Autodesk Inventor part; units mm, degrees
ref_plane "YZ Plane" through (0, 0, 0) normal (1, 0, 0) x (0, 1, 0)
ref_plane "XZ Plane" through (0, 0, 0) normal (0, 1, 0) x (-1, 0, 0)
ref_plane "XY Plane" through (0, 0, 0) normal (0, 0, 1) x (1, 0, 0)
sketch "スケッチ1" plane through (0, 0, 0) normal (0, 0, 1) x (1, 0, 0)
  line L0 (0, 0) -> (0, 3)
  line L1 (0, 3) -> (0.2, 3)
  line L2 (0.2, 3) -> (1.7, 1.5)
  line L3 (1.7, 1.5) -> (7.7, 1.5)
  line L4 (7.7, 1.5) -> (7.7, 0)
  line L5 (0, 0) -> (7.7, 0)
  dimension "d0" = 45
  dimension "d1" = 3
  dimension "d2" = 1.7
  dimension "d3" = 1.5
  dimension "d4" = 6
revolve "回転1" add sketch "スケッチ1" angle 360 about axis through (0, 0, 0) along (1, 0, 0)
thread "ねじ1"
sketch "スケッチ2" plane through (0, 0, 0) normal (-1, 0, 0) x (0, 0, 1)
  line L0 (0.5774, 1) -> (1.1547, 0)
  line L1 (1.1547, 0) -> (0.5774, -1)
  line L2 (0.5774, -1) -> (-0.5774, -1)
  line L3 (-0.5774, -1) -> (-1.1547, 0)
  line L4 (-1.1547, 0) -> (-0.5774, 1)
  line L5 (-0.5774, 1) -> (0.5774, 1)
  circle A0 centre (0, 0) radius 1.1547
  point P0 (0, 0)
  point P1 (0, 0)
  dimension "d8" = 2
extrude "押し出し1" cut sketch "スケッチ2" against normal blind 1.2 contours L0 L1 L2 L3 L4 L5
chamfer "面取り1" distance 0.05 angle 45 6 edges at (0, -0.5, -0.866) (0, 0.5, -0.866) (0, 1, 0) (0, 0.5, 0.866) (0, -1, 0) (0, -0.5, 0.866)
chamfer "面取り2" distance 0.15 angle 45 1 edges at (7.7, -1.5, 0)
properties part number "ネジ皿M3L6" material "鋼、高強度、低合金"
Check sheet for the modelled part. Datum: model origin and axes. Units: mm. A direction names the side the tool comes from. Coordinates: 2 decimals unless noted, no trailing zeros. Write each loop counter-clockwise with the first axis right and the second up, starting at its lowest first coordinate (ties: lowest second). Pieces come first, ordered by that corner, then holes. Notation, with made-up numbers: M -10,29.25 L 47,29.25 A9 ccw 47,40.25 Z; hole C 74,26.25 d7. An arc over 180 degrees is marked long. Use one line per item in the form item = value.
Item 1: Gauge pin test, flat ends, axial feed: pin 1 Ø0.6 at (x, z) = (1, -0.5) entering from -Y; pin 2 Ø1.5 at (x, z) = (3.5, -2) entering from +Y; pin 3 Ø2 at (x, y) = (2, 0.5) entering from +Z; pin 4 Ø1 at (y, z) = (-0.5, -0.5) entering from -X. Record the tip position at first contact, or that the pin passes through.
Answer below:
pin_1 = -2.45
pin_2 = 0.83
pin_3 = 2.16
pin_4 = 0
Item 2: Sectioned sample at A-A, the plane x = 5.25. Record the cut outline in (y, z).
Answer below:
outline = C 0,0 d3
Item 3: Material ranges on L1, parallel to X at y = 0.5, z = -0.25; L2, parallel to Y at x = 4.75, z = -0.05, recorded low to high. Write a range as from..to.
Answer below:
L1 = 1.2..7.7
L2 = -1.5..1.5
Item 4: Set-up check for faces 1 (the face through (0.62, -0.49, 0.87)), 2 (the face through (0, 1.3, 0)): record each of +Z, -Z, +X, -X, +Y, -Y from which the full face is reachable in a straight line by a thin tool's end or side.
Answer below:
face_1 = -X
face_2 = +Z, -Z, -X, +Y, -Y
Item 5: Release check for a two-part mould opening along Z. For faces 3 (the face through (0.62, -0.51, -0.86)), 4 (the face through (7.7, 0, 0)), 5 (the face through (4.67, -1.5, 0.07)) record: pulls with the +Z half, pulls with the -Z half, needs draft (parallel to the pull), parting line crosses it, or undercut.
Answer below:
face_3 = undercut
face_4 = needs draft
face_5 = parting line crosses it
